```python
from build123d import *

# Parameters (mm, degrees)
ESQUISSE1_R             = 24.5
ESQUISSE1_R_2           = 21.5
BOSS_EXTRU_1_DEPTH      = 65.3
ESQUISSE2_R             = 21.5
ESQUISSE2_R_2           = 14.5
BOSS_EXTRU_2_DEPTH      = 3
ESQUISSE3_R             = 1.65
ENL_V_MAT_EXTRU_1_DEPTH = 3
ESQUISSE4_W             = 19
ESQUISSE4_H             = 5.738367338
ENL_V_MAT_EXTRU_2_DEPTH = 23
ESQUISSE5_W             = 68.3
ESQUISSE5_H             = 3
BOSS_EXTRU_3_DEPTH      = 17
ESQUISSE6_W             = 68.3
ESQUISSE6_H             = 3
BOSS_EXTRU_4_DEPTH      = 17
ESQUISSE7_R             = 2
ENL_V_MAT_EXTRU_3_DEPTH = 10
ESQUISSE9_R             = 2
ENL_V_MAT_EXTRU_4_DEPTH = 10
ESQUISSE10_R            = 3.5
ENL_V_MAT_EXTRU_5_DEPTH = 1
ESQUISSE11_R            = 2.75
ENL_V_MAT_EXTRU_6_DEPTH = 8
ESQUISSE12_W            = 17
ESQUISSE12_H            = 3
ENL_V_MAT_EXTRU_7_DEPTH = 74


with BuildPart() as part:
    # Esquisse1 → Boss.-Extru.1 (new body)
    with BuildSketch(Plane.XY):
        Circle(ESQUISSE1_R)
        Circle(ESQUISSE1_R_2, mode=Mode.SUBTRACT)
        with BuildLine():
            Line((-24.5, 0), (-24.5, -24.5))
            Line((-24.5, -24.5), (-6e-09, -24.5))
            ThreePointArc((-6e-09, -24.5), (-17.324116141, -17.324116137), (-24.5, 0))
        make_face()
        with BuildLine():
            ThreePointArc((24.5, 0), (17.324116137, -17.324116141), (-6e-09, -24.5))
            Line((-6e-09, -24.5), (24.5, -24.5))
            Line((24.5, -24.5), (24.5, 0))
        make_face()
    extrude(amount=BOSS_EXTRU_1_DEPTH)

    # Esquisse2 → Boss.-Extru.2 (add)
    with BuildSketch(Plane(origin=(0, 0, 0), x_dir=(-1, 0, 0), z_dir=(0, 0, -1))):
        with BuildLine():
            ThreePointArc((24.5, 0), (0, 24.5), (-24.5, 0))
            ThreePointArc((-24.5, 0), (-17.324116141, -17.324116137), (-6e-09, -24.5))
            ThreePointArc((-6e-09, -24.5), (17.324116137, -17.324116141), (24.5, 0))
        make_face()
        with Locations(Location((0, 0, 0), (0, 0, 180))):
            Circle(ESQUISSE2_R, mode=Mode.SUBTRACT)
        with Locations(Location((0, 0, 0), (0, 0, 180))):
            Circle(ESQUISSE2_R)
        Circle(ESQUISSE2_R_2, mode=Mode.SUBTRACT)
        with BuildLine():
            ThreePointArc((-6e-09, -24.5), (-17.324116141, -17.324116137), (-24.5, 0))
            Line((-24.5, 0), (-24.5, -24.5))
            Line((-24.5, -24.5), (-6e-09, -24.5))
        make_face()
        with BuildLine():
            Line((24.5, -24.5), (24.5, 0))
            ThreePointArc((24.5, 0), (17.324116137, -17.324116141), (-6e-09, -24.5))
            Line((-6e-09, -24.5), (24.5, -24.5))
        make_face()
    extrude(amount=BOSS_EXTRU_2_DEPTH)

    # Esquisse3 → Enlèv. mat.-Extru.1 (cut)
    with BuildSketch(Plane(origin=(0, 0, -3), x_dir=(-1, 0, 0), z_dir=(0, 0, -1))):
        with Locations((-17.5, 0)):
            Circle(ESQUISSE3_R)
        with Locations((17.5, 0)):
            Circle(ESQUISSE3_R)
        with Locations((0, 17.5)):
            Circle(ESQUISSE3_R)
        with Locations((0, -17.5)):
            Circle(ESQUISSE3_R)
    extrude(amount=-ENL_V_MAT_EXTRU_1_DEPTH, mode=Mode.SUBTRACT)

    # Esquisse4 → Enlèv. mat.-Extru.2 (cut)
    with BuildSketch(Plane.XY.offset(65.3)):
        with Locations((0, 22.156485191)):
            Rectangle(ESQUISSE4_W, ESQUISSE4_H)
    extrude(amount=-ENL_V_MAT_EXTRU_2_DEPTH, mode=Mode.SUBTRACT)

    # Esquisse5 → Boss.-Extru.3 (add)
    with BuildSketch(Plane.ZY.offset(24.5)):
        with Locations((31.15, -23)):
            Rectangle(ESQUISSE5_W, ESQUISSE5_H)
    extrude(amount=BOSS_EXTRU_3_DEPTH)

    # Esquisse6 → Boss.-Extru.4 (add)
    with BuildSketch(Plane(origin=(24.5, 0, 0), x_dir=(0, 0, -1), z_dir=(1, 0, 0))):
        with Locations((-31.15, -23)):
            Rectangle(ESQUISSE6_W, ESQUISSE6_H)
    extrude(amount=BOSS_EXTRU_4_DEPTH)

    # Esquisse7 → Enlèv. mat.-Extru.3 (cut)
    with BuildSketch(Plane(origin=(0, -21.5, 0), x_dir=(1, 0, 0), z_dir=(0, 1, 0))):
        with Locations(Location((-33, -7, 0), (0, 0, 270))):
            Circle(ESQUISSE7_R)
        with Locations(Location((-33, -55.3, 0), (0, 0, 270))):
            Circle(ESQUISSE7_R)
    extrude(amount=-ENL_V_MAT_EXTRU_3_DEPTH, mode=Mode.SUBTRACT)

    # Esquisse9 → Enlèv. mat.-Extru.4 (cut)
    with BuildSketch(Plane(origin=(0, -21.5, 0), x_dir=(1, 0, 0), z_dir=(0, 1, 0))):
        with Locations(Location((33, -7, 0), (0, 0, 270))):
            Circle(ESQUISSE9_R)
        with Locations(Location((33, -55.3, 0), (0, 0, 270))):
            Circle(ESQUISSE9_R)
    extrude(amount=-ENL_V_MAT_EXTRU_4_DEPTH, mode=Mode.SUBTRACT)

    # Esquisse10 → Enlèv. mat.-Extru.5 (cut)
    with BuildSketch(Plane.XZ.offset(24.5)):
        with Locations(Location((-19.5, 55.3, 0), (0, 0, 270))):
            Circle(ESQUISSE10_R)
        with Locations(Location((19.5, 55.3, 0), (0, 0, 90))):
            Circle(ESQUISSE10_R)
        with Locations(Location((19.5, 7, 0), (0, 0, 270))):
            Circle(ESQUISSE10_R)
        with Locations(Location((-19.5, 7, 0), (0, 0, 90))):
            Circle(ESQUISSE10_R)
    extrude(amount=-ENL_V_MAT_EXTRU_5_DEPTH, mode=Mode.SUBTRACT)

    # Esquisse11 → Enlèv. mat.-Extru.6 (cut)
    with BuildSketch(Plane.XZ.offset(24.5)):
        with Locations(Location((-19.5, 55.3, 0), (0, 0, 270))):
            Circle(ESQUISSE11_R)
        with Locations(Location((19.5, 55.3, 0), (0, 0, 90))):
            Circle(ESQUISSE11_R)
        with Locations(Location((19.5, 7, 0), (0, 0, 270))):
            Circle(ESQUISSE11_R)
        with Locations(Location((-19.5, 7, 0), (0, 0, 90))):
            Circle(ESQUISSE11_R)
    extrude(amount=-ENL_V_MAT_EXTRU_6_DEPTH, mode=Mode.SUBTRACT)

    # Esquisse12 → Enlèv. mat.-Extru.7 (cut)
    with BuildSketch(Plane(origin=(0, 0, -3), x_dir=(-1, 0, 0), z_dir=(0, 0, -1))):
        with Locations((-33, -23)):
            Rectangle(ESQUISSE12_W, ESQUISSE12_H)
        with Locations((33, -23)):
            Rectangle(ESQUISSE12_W, ESQUISSE12_H)
    extrude(amount=-ENL_V_MAT_EXTRU_7_DEPTH, mode=Mode.SUBTRACT)


solid = part.part
```
Verification items for the finished model (mm, model axes). A direction names the side the tool comes from. Coordinates: 2 decimals unless noted, no trailing zeros. Write each loop counter-clockwise with the first axis right and the second up, starting at its lowest first coordinate (ties: lowest second). Pieces come first, ordered by that corner, then holes. Notation, with made-up numbers: (88.5, 54) - (108.5, 54) arc R5 ccw to (108.5, 61) - close; hole circle Ø7 at (-37.5, -7). An arc over 180 degrees is marked (long way). Write item = value, one per line.
Q1. Material ranges on L1, parallel to X at y = -23.7, z = 7; L2, parallel to Y at x = 0, z = -1.1; L3, parallel to Y at x = 16, z = 41, recorded low to high. Write a range as from..to.
Answer:
L1 = -24.5..-23, -16..16, 23..24.5
L2 = -24.5..-19.15, -15.85..-14.5, 14.5..15.85, 19.15..24.5
L3 = -24.5..-14.36, 14.36..18.55
Q2. Go/stop test with flat-tipped pins: pin 1 Ø6 at (y, z) = (19.5, 57) entering from -X; pin 2 Ø2.5 at (x, y) = (0, 17.5) entering from -Z; pin 3 Ø1.6 at (y, z) = (21.5, 48.5) entering from -X; pin 4 Ø10 at (x, z) = (-12.5, 56.5) entering from +Y. Record where each tip stops, or that it passes through.
Answer:
pin_1 = -18.11
pin_2 = through
pin_3 = -13.11
pin_4 = 22.58
Q3. Cross-section at C-C (x = 0). Enter the section's corners in (y, z).
Answer:
outline = (-24.5, -3) - (-19.15, -3) - (-19.15, 0) - (-21.5, 0) - (-21.5, 65.3) - (-24.5, 65.3) - close; (-15.85, -3) - (-14.5, -3) - (-14.5, 0) - (-15.85, 0) - close; (14.5, -3) - (15.85, -3) - (15.85, 0) - (14.5, 0) - close; (19.15, -3) - (24.5, -3) - (24.5, 42.3) - (21.5, 42.3) - (21.5, 0) - (19.15, 0) - close
Q4. Access from +Z, -Z, +X, -X, +Y, -Y to the whole of each face (thin tool, end or side, straight path). Record for faces 1 (the face through (-6.691, -12.864, -1.479)), 2 (the face through (0, 23, 42.3)), 3 (the face through (-4.66, -20.99, 32.19)), 4 (the face through (-20, -16.5, 7)).
Answer:
face_1 = +Z, -Z
face_2 = +Z, +Y
face_3 = +Z
face_4 = -Y
Q5. Cross-section at A-A (y = -17.5). Enter the section's corners in (x, z).
Answer:
outline = (-24.5, -3) - (-1.65, -3) - (-1.65, 0) - (-12.49, 0) - (-12.49, 65.3) - (-24.5, 65.3) - close; (1.65, -3) - (24.5, -3) - (24.5, 65.3) - (12.49, 65.3) - (12.49, 0) - (1.65, 0) - close; hole circle Ø5.5 at (-19.5, 7); hole circle Ø5.5 at (-19.5, 55.3); hole circle Ø5.5 at (19.5, 7); hole circle Ø5.5 at (19.5, 55.3)
Q6. Mould release check, pull along Z, two halves, no side actions. Record for faces 5 (the face through (18.67, -20.05, 57.92)), 6 (the face through (-9.5, 21, 54)), 7 (the face through (0, 15, 0)), 8 (the face through (11, -11, -3)): released by +Z, released by -Z, zero draft, split by the parting line, or undercut.
Answer:
face_5 = undercut
face_6 = zero draft
face_7 = released by +Z
face_8 = released by -Z
Q7. Cross-section at D-D (y = 10.5). Enter the section's corners in (x, z), plus the area to 3 significant figures.
Answer:
outline = (-22.14, -3) - (-10, -3) - (-10, 0) - (-18.76, 0) - (-18.76, 65.3) - (-22.14, 65.3) - close; (10, -3) - (22.14, -3) - (22.14, 65.3) - (18.76, 65.3) - (18.76, 0) - (10, 0) - close
area = 513 mm²
Q8. Cross-section at B-B (z = 7). Enter the section's corners in (x, y), plus the area to 3 significant figures.
Answer:
outline = (-24.5, -24.5) - (-23, -24.5) - (-23, -23.5) - (-22.25, -23.5) - (-22.25, -16.5) - (-16.75, -16.5) - (-16.75, -23.5) - (-16, -23.5) - (-16, -24.5) - (16, -24.5) - (16, -23.5) - (16.75, -23.5) - (16.75, -16.5) - (22.25, -16.5) - (22.25, -23.5) - (23, -23.5) - (23, -24.5) - (24.5, -24.5) - (24.5, 0) arc R24.5 ccw to (-24.5, 0) - close; hole circle Ø43 at (0, 0)
area = 600 mm²
